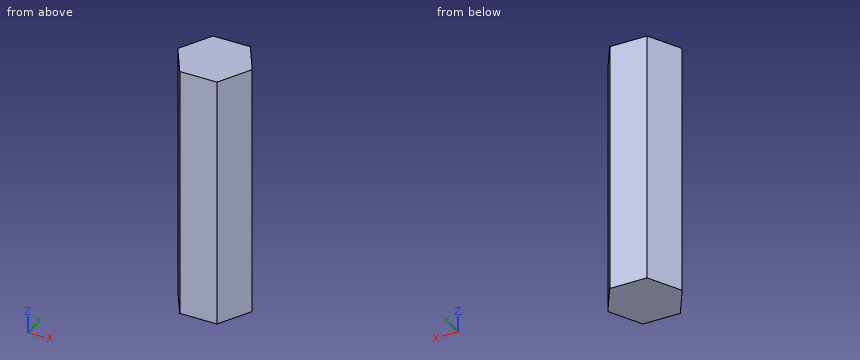
Autodesk Inventor part; units mm, degrees
ref_plane "YZ Plane" through (0, 0, 0) normal (1, 0, 0) x (0, 1, 0)
ref_plane "XZ Plane" through (0, 0, 0) normal (0, 1, 0) x (-1, 0, 0)
ref_plane "XY Plane" through (0, 0, 0) normal (0, 0, 1) x (1, 0, 0)
sketch "Sketch1" plane through (0, 0, 0) normal (0, 0, 1) x (1, 0, 0)
  line L0 (7.3323, 0) -> (3.6662, -6.35)
  line L1 (3.6662, -6.35) -> (-3.6662, -6.35)
  line L2 (-3.6662, -6.35) -> (-7.3323, 0)
  line L3 (-7.3323, 0) -> (-3.6662, 6.35)
  line L4 (-3.6662, 6.35) -> (3.6662, 6.35)
  line L5 (3.6662, 6.35) -> (7.3323, 0)
  point P0 (0, 0)
  point P1 (0, 0)
  dimension "d0" = 12.7
extrude "Extrusion1" add sketch "Sketch1" against normal blind 50.8
properties part number "hexShaft"
Can you work these out from the model? Positions are in its coordinate system, mm. Round coordinates to 2 decimals unless told otherwise and drop trailing zeros. Loops run counter-clockwise (first coordinate to the right, second up) from the corner with the lowest first, then second, coordinate; pieces in that order, holes last. Notation, with made-up numbers: (45.5, 24) - (76.5, 24) arc R16 ccw to (76.5, 33) - close; hole circle Ø8 at (69.25, 82). An arc over 180 degrees is marked (long way). Use CSV: the item, a comma, the result in double quotes. Start each with the question number.
1) If we section it at C-C on x = 4.25: Write out the boundary of the cut face in (y, z).
2) If we section it at A-A on z = -46: Write out the boundary of the cut face in (x, y).
3) If we section it at B-B on y = -3.25: Write out the boundary of the cut face in (x, z), plus the area to 3 significant figures.
4) Please list where these lines run through material, in increasing order: probe 1 along X at (y, z) = (4.75, -45); probe 2 along X at (y, z) = (-3.25, -16); probe 3 along Y at (x, z) = (4.75, -45.5). Write a range as [from, to].
Geometry results:
1,outline,"(-5.34, -50.8) - (5.34, -50.8) - (5.34, 0) - (-5.34, 0) - close"
2,outline,"(-7.33, 0) - (-3.67, -6.35) - (3.67, -6.35) - (7.33, 0) - (3.67, 6.35) - (-3.67, 6.35) - close"
3,outline,"(-5.46, -50.8) - (5.46, -50.8) - (5.46, 0) - (-5.46, 0) - close"
3,area,"554 mm2"
4,probe 1,"x = [-4.59, 4.59]"
4,probe 2,"x = [-5.46, 5.46]"
4,probe 3,"y = [-4.47, 4.47]"
